Check sheet for the drawn part. Datum: minimum x, y, z corner. Units: mm. A direction names the side the tool comes from. Give positions to 0.01 mm unless a question says otherwise; leave off trailing zeros. Write each loop counter-clockwise with the first axis right and the second up, starting at its lowest first coordinate (ties: lowest second). Pieces come first, ordered by that corner, then holes.
(1) Cross-section at D-D (x = 39.5). Count the separate pieces of the cut face and the enclosed holes in it.
(2) Thickness scan on line 1 along Y through (x, z) = (35.5, 4.25); line 2 along X through (y, z) = (7.75, 11); line 3 along X through (y, z) = (15, 11.5). Record the ranges inside material, lowest first.
(3) Cross-section at A-A (x = 28). Record the boundary of the cut face in (y, z).
(4) Depth check by flat-ended pin: P1, Ø6, axis at y = 16, z = 8, coming from the -X side; P2, Ø1, axis at x = 22.5, z = 13, coming from the -Y side; P3, Ø4.5, axis at y = 18, z = 5.5, coming from the -X side; P4, Ø4, axis at x = 39, z = 8.5, coming from the -Y side. Enter the tip coordinate at first touch or a pass-through.
(5) Mould release check, pull along Z, two halves, no side actions. Record for the marked faces 1, 2, 3 and 4: +Z half, -Z half, draft (parallel to the pull), parting line (faces both ways), or undercut.
(6) Cross-section at C-C (y = 11). Record the boundary of the cut face in (x, z).
(7) Cross-section at B-B (y = 18.25). Record the boundary of the cut face in (x, z), and give its area (3 significant figures).
(8) Tool access check on the marked faces 5, 6, 7, 8 and 9. Record the directions out of +Z, -Z, +X, -X, +Y, -Y that give a thin tool (end or side, any length) a straight path to the whole face; none if there is none.
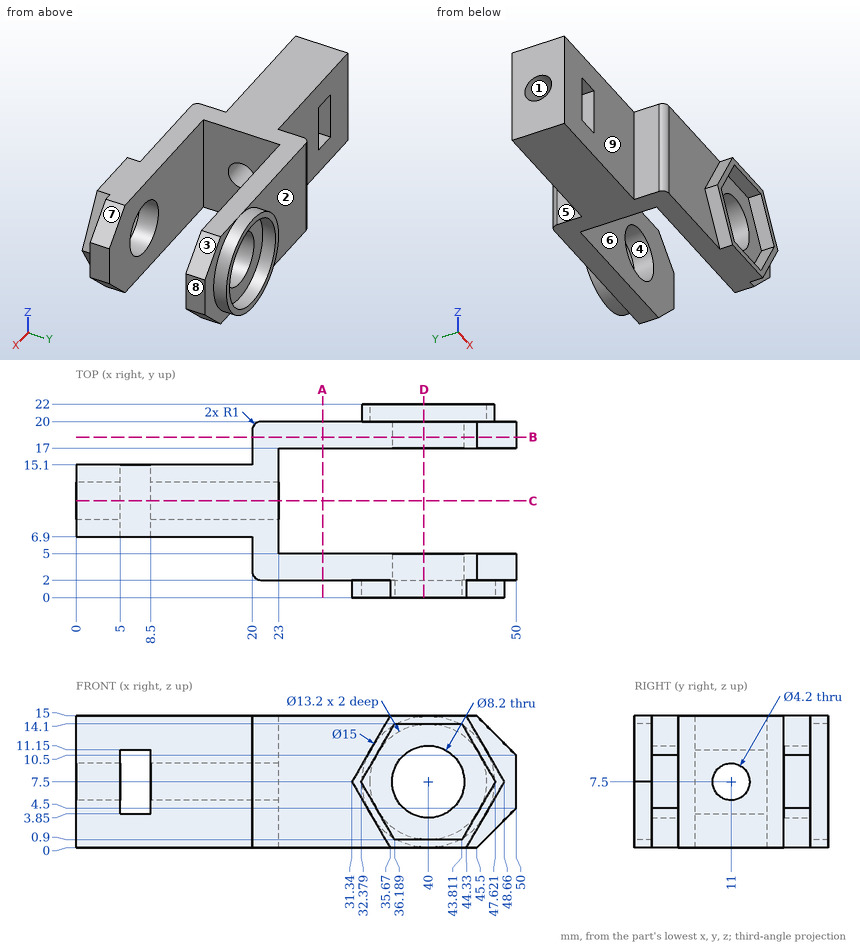
Reply:
1. separate pieces: 4
1. enclosed holes: 0
2. line 1: y = 2 to 5, 17 to 20
2. line 2: x = 0 to 5, 8.5 to 23
2. line 3: x = 0 to 23
3. outline: (2, 0) - (5, 0) - (5, 15) - (2, 15) - close; (17, 0) - (20, 0) - (20, 15) - (17, 15) - close
4. P1: stops at x = 0
4. P2: stops at y = 2
4. P3: stops at x = 20
4. P4: passes through
5. face 1: undercut
5. face 2: draft
5. face 3: +Z half
5. face 4: undercut
6. outline: (0, 0) - (23, 0) - (23, 5.4) - (8.5, 5.4) - (8.5, 3.85) - (5, 3.85) - (5, 5.4) - (0, 5.4) - close; (0, 9.6) - (5, 9.6) - (5, 11.15) - (8.5, 11.15) - (8.5, 9.6) - (23, 9.6) - (23, 15) - (0, 15) - close
7. outline: (20, 0) - (45.5, 0) - (50, 4.5) - (50, 10.5) - (45.5, 15) - (20, 15) - close; hole circle Ø8.2 at (40, 7.5)
7. area: 377 mm2
8. face 5: +Z, -Z, -X, +Y
8. face 6: +Z, -Z, +X
8. face 7: +Z, +X, +Y, -Y
8. face 8: +Z, -Z, +X, +Y, -Y
8. face 9: +Z, -Z, -X, -Y
